Read the model definition and answer for the solid it produces. Units are mm, in the model's axes. Coordinates: 2 decimals unless noted, no trailing zeros. Order: outer loops, then holes, each group sorted by start corner. A loop starts at its lowest first (then second) coordinate and runs counter-clockwise, first axis right, second up. Notation, with made-up numbers: (-36, -29) - (-14, -29) arc R8 cw to (-14, -24) - close; hole circle Ø2 at (47.5, -7.75). An arc over 180 degrees is marked (long way). Write item = value, one per line.
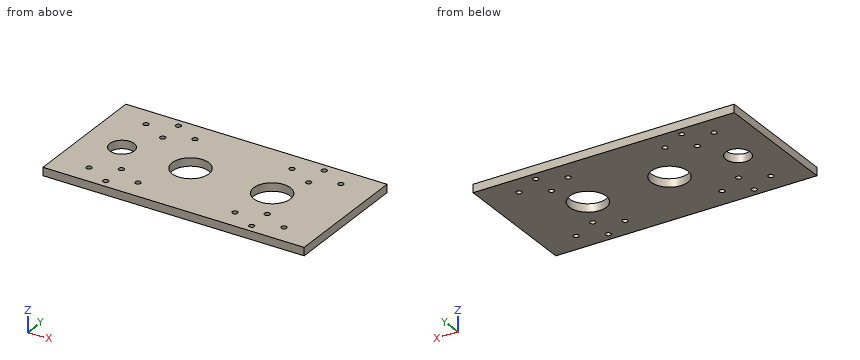
from build123d import *

# Parameters (mm, degrees)
SKETCH1_W               = 203.2
SKETCH1_H               = 101.6
BOSS_EXTRUDE1_DEPTH     = 6.35
SKETCH3_R               = 14.2875
SKETCH3_R_2             = 9.525
CUT_EXTRUDE2_DEPTH      = 6.35
SKETCH5_R               = 2.0828
CUT_EXTRUDE3_DEPTH      = 228.273233136
MIRROR2_COPY_1_SKETCH_R = 2.0828
MIRROR2_COPY_1_DEPTH    = 228.273233136


with BuildPart() as part:
    # Sketch1 → Boss-Extrude1 (new body)
    with BuildSketch(Plane.XY):
        with Locations((101.6, 50.8)):
            Rectangle(SKETCH1_W, SKETCH1_H)
    extrude(amount=BOSS_EXTRUDE1_DEPTH)

    # Sketch3 → Cut-Extrude2 (cut)
    with BuildSketch(Plane.XY.offset(6.35)):
        with Locations((82.55, 50.8)):
            Circle(SKETCH3_R)
        with Locations(Location((146.05, 50.8, 0), (0, 0, 180))):
            Circle(SKETCH3_R)
        with Locations((29.21, 50.8)):
            Circle(SKETCH3_R_2)
    extrude(amount=-CUT_EXTRUDE2_DEPTH, mode=Mode.SUBTRACT)

    # Sketch5 → Cut-Extrude3 (cut, through all)
    with BuildSketch(Plane.XY.offset(6.35)):
        with Locations((139.319, 85.725)):
            Circle(SKETCH5_R)
        with Locations((158.369, 95.25)):
            Circle(SKETCH5_R)
        with Locations((158.369, 76.2)):
            Circle(SKETCH5_R)
        with Locations((177.419, 85.725)):
            Circle(SKETCH5_R)
    cut_extrude3 = extrude(amount=-CUT_EXTRUDE3_DEPTH, mode=Mode.SUBTRACT)

    # Mirror1: Cut-Extrude3 across plane
    add(cut_extrude3.mirror(Plane.ZX.offset(50.8)), mode=Mode.SUBTRACT)

    # Mirror2: Cut-Extrude3 across plane
    add(cut_extrude3.mirror(Plane(origin=(101.6, 0, 0), x_dir=(0, 0, 1), z_dir=(1, 0, 0))), mode=Mode.SUBTRACT)

    # Mirror2 copy 1 sketch → Mirror2 copy 1 (cut, through all)
    with BuildSketch(Plane(origin=(203.2, 101.6, 6.35), x_dir=(-1, 0, 0), z_dir=(0, 0, 1))):
        with Locations((139.319, 85.725)):
            Circle(MIRROR2_COPY_1_SKETCH_R)
        with Locations((158.369, 95.25)):
            Circle(MIRROR2_COPY_1_SKETCH_R)
        with Locations((158.369, 76.2)):
            Circle(MIRROR2_COPY_1_SKETCH_R)
        with Locations((177.419, 85.725)):
            Circle(MIRROR2_COPY_1_SKETCH_R)
    extrude(amount=-MIRROR2_COPY_1_DEPTH, mode=Mode.SUBTRACT)


solid = part.part
1) The part is cut by section B-B (y = 76.2). Determine the outline of the cut face in (x, z).
Returned:
outline = (0, 0) - (42.75, 0) - (42.75, 6.35) - (0, 6.35) - close; (46.91, 0) - (156.29, 0) - (156.29, 6.35) - (46.91, 6.35) - close; (160.45, 0) - (203.2, 0) - (203.2, 6.35) - (160.45, 6.35) - close
2) The part is cut by section A-A (x = 146.05). Determine the outline of the cut face in (y, z), and give its area (3 significant figures).
Returned:
outline = (0, 0) - (36.51, 0) - (36.51, 6.35) - (0, 6.35) - close; (65.09, 0) - (101.6, 0) - (101.6, 6.35) - (65.09, 6.35) - close
area = 464 mm^2
3) The part is cut by section C-C (z = 1.5). Count the separate pieces of the cut face and the enclosed holes in it, and give its area (3 significant figures).
Returned:
separate_pieces = 1
enclosed_holes = 19
area = 18,900 mm^2
4) A flat-ended cylindrical pin translates along its axis: pin 1 Ø3.5 at (x, y) = (177.419, 85.725) entering from +Z. Find the tip coordinate at first contact, or state that the pin passes through.
Returned:
pin_1 = through
5) Straight lines are drawn through the part: line 1 along X through (y, z) = (6.5, 6); line 2 along X through (y, z) = (75, 3); line 3 along X through (y, z) = (55, 5.5). For each, find the intervals that lie inside material, in ascending order. Write a range as from..to.
Returned:
line_1 = 0..42.75, 46.91..156.29, 160.45..203.2
line_2 = 0..43.13, 46.53..156.67, 160.07..203.2
line_3 = 0..20.66, 37.76..68.89, 96.21..132.39, 159.71..203.2
